Can you work these out from the model? Positions are in its coordinate system, mm. Face numbers are marked on the shaded views. A direction names the side the tool comes from. Coordinates: 2 decimals unless noted, no trailing zeros. Order: outer loops, then holes, each group sorted by start corner. A loop starts at its lowest first (then second) coordinate and runs counter-clockwise, first axis right, second up.
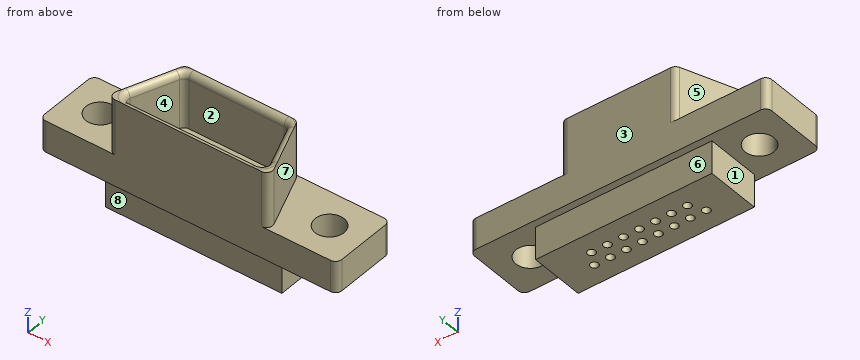
```python
from build123d import *

# Parameters (mm, degrees)
SKETCH_1_W          = 23.6
SKETCH_1_H          = 5.4
SKETCH_1_R          = 1.15
EXTRUDE_1_DEPTH     = 2.5
FILLET_1_R          = 0.5
FILLET_2_R          = 0.5
SKETCH_3_W          = 14
SKETCH_3_H          = 4.3
EXTRUDE_2_DEPTH     = 2.6
SKETCH_4_R          = 0.31
CUT_EXTRUDE_1_DEPTH = 4.5
EXTRUDE_3_DEPTH     = 4.4
FILLET_3_R          = 0.5


with BuildPart() as part:
    # 草图1 → 凸台-拉伸1 (new body)
    with BuildSketch(Plane.XY):
        Rectangle(SKETCH_1_W, SKETCH_1_H)
        with Locations((-9.1, 0)):
            Circle(SKETCH_1_R, mode=Mode.SUBTRACT)
        with Locations(Location((9.1, 0, 0), (0, 0, 180))):
            Circle(SKETCH_1_R, mode=Mode.SUBTRACT)
    extrude(amount=EXTRUDE_1_DEPTH)

    # 圆角1
    fillet_1_edges = [part.edges().sort_by_distance(p)[0] for p in [
        (-11.8, 2.7, 1.25),
    ]]
    fillet(fillet_1_edges, radius=FILLET_1_R)

    # 圆角2
    fillet_2_edges = [part.edges().sort_by_distance(p)[0] for p in [
        (11.8, 2.7, 1.25),
        (11.8, -2.7, 1.25),
        (-11.8, -2.7, 1.25),
    ]]
    fillet(fillet_2_edges, radius=FILLET_2_R)

    # 草图3 → 凸台-拉伸2 (add)
    with BuildSketch(Plane(origin=(0, 0, 0), x_dir=(-1, 0, 0), z_dir=(0, 0, -1))):
        Rectangle(SKETCH_3_W, SKETCH_3_H)
    extrude(amount=EXTRUDE_2_DEPTH)

    # 草图4 → 切除-拉伸1 (cut)
    with BuildSketch(Plane(origin=(0, 0, -2.6), x_dir=(-1, 0, 0), z_dir=(0, 0, -1))):
        with Locations((0, 0.55)):
            Circle(SKETCH_4_R)
        with Locations((1.27, 0.55)):
            Circle(SKETCH_4_R)
        with Locations((2.54, 0.55)):
            Circle(SKETCH_4_R)
        with Locations((3.81, 0.55)):
            Circle(SKETCH_4_R)
        with Locations(Location((-3.81, 0.55, 0), (0, 0, 180))):
            Circle(SKETCH_4_R)
        with Locations(Location((-2.54, 0.55, 0), (0, 0, 180))):
            Circle(SKETCH_4_R)
        with Locations(Location((-1.27, 0.55, 0), (0, 0, 180))):
            Circle(SKETCH_4_R)
        with Locations(Location((-4.445, -0.55, 0), (0, 0, 180))):
            Circle(SKETCH_4_R)
        with Locations(Location((-3.175, -0.55, 0), (0, 0, 180))):
            Circle(SKETCH_4_R)
        with Locations(Location((-1.905, -0.55, 0), (0, 0, 180))):
            Circle(SKETCH_4_R)
        with Locations(Location((-0.635, -0.55, 0), (0, 0, 180))):
            Circle(SKETCH_4_R)
        with Locations(Location((0.635, -0.55, 0), (0, 0, 180))):
            Circle(SKETCH_4_R)
        with Locations(Location((1.905, -0.55, 0), (0, 0, 180))):
            Circle(SKETCH_4_R)
        with Locations(Location((3.175, -0.55, 0), (0, 0, 180))):
            Circle(SKETCH_4_R)
        with Locations(Location((4.445, -0.55, 0), (0, 0, 180))):
            Circle(SKETCH_4_R)
    extrude(amount=-CUT_EXTRUDE_1_DEPTH, mode=Mode.SUBTRACT)

    # 草图5 → 凸台-拉伸3 (add)
    with BuildSketch(Plane.XY.offset(2.5)):
        with BuildLine():
            Line((-4.153912025, 2.7), (4.094589559, 2.7))
            ThreePointArc((4.094589559, 2.7), (4.376736154, 2.612787232), (4.560455607, 2.381573196))
            Line((4.560455607, 2.381573196), (6.275373584, -2.018426804))
            ThreePointArc((6.275373584, -2.018426804), (6.222294768, -2.482146595), (5.809507536, -2.7))
            Line((5.809507536, -2.7), (-5.809507536, -2.7))
            ThreePointArc((-5.809507536, -2.7), (-6.220628978, -2.484568375), (-6.277476178, -2.02391664))
            Line((-6.277476178, -2.02391664), (-4.621880667, 2.37608336))
            ThreePointArc((-4.621880667, 2.37608336), (-4.4384804, 2.611121442), (-4.153912025, 2.7))
        make_face()
        with BuildLine():
            Line((-3.807824049, 2.2), (3.752831659, 2.2))
            ThreePointArc((3.752831659, 2.2), (4.034978254, 2.112787232), (4.218697707, 1.881573196))
            Line((4.218697707, 1.881573196), (5.543861598, -1.518426804))
            ThreePointArc((5.543861598, -1.518426804), (5.490782782, -1.982146595), (5.07799555, -2.2))
            Line((5.07799555, -2.2), (-5.087147854, -2.2))
            ThreePointArc((-5.087147854, -2.2), (-5.498269295, -1.984568375), (-5.555116496, -1.52391664))
            Line((-5.555116496, -1.52391664), (-4.275792692, 1.87608336))
            ThreePointArc((-4.275792692, 1.87608336), (-4.092392424, 2.111121442), (-3.807824049, 2.2))
        make_face(mode=Mode.SUBTRACT)
    extrude(amount=EXTRUDE_3_DEPTH)

    # 圆角3
    fillet_3_edges = [part.edges().sort_by_distance(p)[0] for p in [
        (5.490782782, -1.982146595, 6.9),
        (4.881279653, 0.181573196, 6.9),
        (4.034978254, 2.112787232, 6.9),
        (-0.027496195, 2.2, 6.9),
        (-4.092392424, 2.111121442, 6.9),
        (-4.915454594, 0.17608336, 6.9),
        (-5.498269295, -1.984568375, 6.9),
        (-0.004576152, -2.2, 6.9),
    ]]
    fillet(fillet_3_edges, radius=FILLET_3_R - 0.0001)  # a hair under: the kernel refuses the full size


solid = part.part
```
1. I'm going to push flat-ended pins straight in: pin 1 (0.8 mm diameter, centred on x = -2, z = -0.5, fed in from -Y); pin 2 (0.8 mm diameter, centred on y = 1, z = -2, fed in from -X). Where does each tip first touch, or does it pass through?
Completed:
pin 1: stops at y = -2.15
pin 2: stops at x = -7
2. Please list where these lines run through material, in increasing order: probe 1 along Y at (x, z) = (1.27, -0.35); probe 2 along Y at (x, z) = (2, 3.75); probe 3 along Z at (x, y) = (-8, 2.4).
Completed:
probe 1: y = -2.15 to 0.24, 0.86 to 2.15
probe 2: y = -2.7 to -2.2, 2.2 to 2.7
probe 3: z = 0 to 2.5
3. On a 3-axis mill with a long thin cutter (end or side, diameter ignored), from which of +Z, -Z, +X, -X, +Y, -Y can I reach the whole of each face in a straight line? I mean the marked faces 5, 6, 7 and 8. Say none if no direction works.
Completed:
face 5: +Z, -X, +Y
face 6: -Z, +X, -X, +Y
face 7: +Z, +X, +Y
face 8: -Z, +X, -X, -Y
4. Imagine slicing it at B-B on x = 9.1. Please give me the cut outline in (y, z).
Completed:
outline: (-2.7, 0) - (-1.15, 0) - (-1.15, 2.5) - (-2.7, 2.5) - close; (1.15, 0) - (2.7, 0) - (2.7, 2.5) - (1.15, 2.5) - close
5. Imagine slicing it at A-A on z = -1.25. Give the number of separate pieces and of enclosed holes in the cut face, then the cut area to 3 significant figures.
Completed:
separate pieces: 1
enclosed holes: 15
area: 55.7 mm2
6. Thinking about a two-plate mould opening in Y: for the marked faces 1, 2, 3 and 4, which applies, pulls with the +Y half, pulls with the -Y half, needs draft (parallel to the pull), parting line crosses it, or undercut?
Completed:
face 1: needs draft
face 2: undercut
face 3: pulls with the +Y half
face 4: undercut
